```python
from build123d import *

# Parameters (mm, degrees)
CROQUIS1_W              = 160
CROQUIS1_H              = 50.8
SALIENTE_EXTRUIR1_DEPTH = 300
CROQUIS2_W              = 160
CROQUIS2_H              = 25.4
SALIENTE_EXTRUIR2_DEPTH = 100
CROQUIS3_R              = 12.5
CORTAR_EXTRUIR1_DEPTH   = 100
CROQUIS4_R              = 18
CORTAR_EXTRUIR2_DEPTH   = 5
CORTAR_EXTRUIR3_START   = -5
CROQUIS5_R              = 18
CORTAR_EXTRUIR3_DEPTH   = 5


with BuildPart() as part:
    # Croquis1 → Saliente-Extruir1 (new, symmetric)
    with BuildSketch(Plane.XY):
        Rectangle(CROQUIS1_W, CROQUIS1_H)
    extrude(amount=SALIENTE_EXTRUIR1_DEPTH, both=True)

    # Croquis2 → Saliente-Extruir2 (add)
    with BuildSketch(Plane(origin=(0, 25.4, 0), x_dir=(1, 0, 0), z_dir=(0, 1, 0))):
        with Locations((0, 287.3)):
            Rectangle(CROQUIS2_W, CROQUIS2_H)
    extrude(amount=SALIENTE_EXTRUIR2_DEPTH)

    # Croquis3 → Cortar-Extruir1 (cut)
    with BuildSketch(Plane.XY.offset(-274.6)):
        with Locations((0, 59.234859244)):
            Circle(CROQUIS3_R)
    extrude(amount=-CORTAR_EXTRUIR1_DEPTH, mode=Mode.SUBTRACT)

    # Croquis4 → Cortar-Extruir2 (cut)
    with BuildSketch(Plane.XY.offset(-274.6)):
        with Locations((0, 59.234859244)):
            Circle(CROQUIS4_R)
    extrude(amount=-CORTAR_EXTRUIR2_DEPTH, mode=Mode.SUBTRACT)

    # Croquis5 → Cortar-Extruir3 (cut)
    with BuildSketch(Plane(origin=(0, 0, -300), x_dir=(-1, 0, 0), z_dir=(0, 0, -1)).offset(CORTAR_EXTRUIR3_START)):
        with Locations(Location((0, 59.234859244, 0), (0, 0, 180))):
            Circle(CROQUIS5_R)
    extrude(amount=CORTAR_EXTRUIR3_DEPTH, mode=Mode.SUBTRACT)


solid = part.part
```
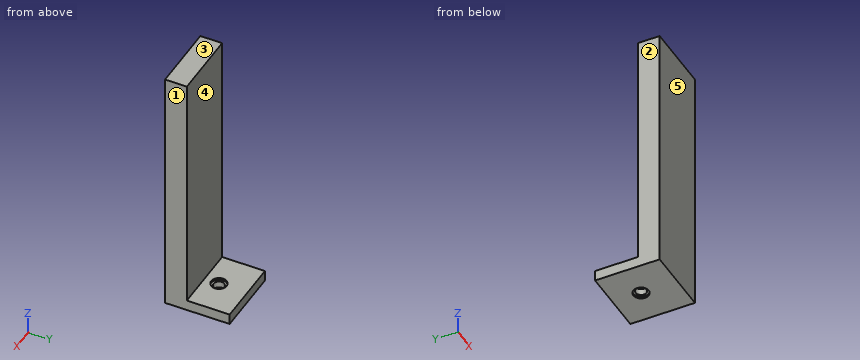
Verification items for the finished model (mm, model axes). Face numbers are marked on the shaded views. A direction names the side the tool comes from. Give positions to 0.01 mm unless a question says otherwise; leave off trailing zeros. Order: outer loops, then holes, each group sorted by start corner. A loop starts at its lowest first (then second) coordinate and runs counter-clockwise, first axis right, second up. Notation, with made-up numbers: (30, -17) -> (79, -17) arc R11 ccw to (79, -13) -> close; hole circle Ø4 at (-8.75, -21). An arc over 180 degrees is marked (long way). Use a Markdown table: item, result.
1) Section check A-A, the plane x = 0. Record the boundary of the cut face in (y, z), then the cut area to 3 significant figures.
Results:
| item | result |
|---|---|
| outline | (-25.4, -300) -> (41.23, -300) -> (41.23, -295) -> (46.73, -295) -> (46.73, -279.6) -> (41.23, -279.6) -> (41.23, -274.6) -> (25.4, -274.6) -> (25.4, 300) -> (-25.4, 300) -> close; (71.73, -295) -> (77.23, -295) -> (77.23, -300) -> (125.4, -300) -> (125.4, -274.6) -> (77.23, -274.6) -> (77.23, -279.6) -> (71.73, -279.6) -> close |
| area | 32,300 mm² |
2) Material ranges on probe 1 along Y at (x, z) = (0, -285.75); probe 2 along Y at (x, z) = (0, -277); probe 3 along Y at (x, z) = (13.5, 67.5), recorded low to high.
Results:
| item | result |
|---|---|
| probe 1 | -25.4 to 46.73, 71.73 to 125.4 |
| probe 2 | -25.4 to 41.23, 77.23 to 125.4 |
| probe 3 | -25.4 to 25.4 |
3) Tool access check on the marked faces 4 and 5. Record the directions out of +Z, -Z, +X, -X, +Y, -Y that give a thin tool (end or side, any length) a straight path to the whole face; none if there is none.
Results:
| item | result |
|---|---|
| face 4 | +Z, +X, -X, +Y |
| face 5 | +Z, -Z, +X, -X, -Y |
4) Section check D-D, the plane z = 167.5. Record the boundary of the cut face in (x, y).
Results:
| item | result |
|---|---|
| outline | (-80, -25.4) -> (80, -25.4) -> (80, 25.4) -> (-80, 25.4) -> close |
5) Section check C-C, the plane y = 100. Record the boundary of the cut face in (x, z).
Results:
| item | result |
|---|---|
| outline | (-80, -300) -> (80, -300) -> (80, -274.6) -> (-80, -274.6) -> close |
6) Mould release check, pull along X, two halves, no side actions. Record for the marked faces 1, 2 and 3: pulls with the +X half, pulls with the -X half, needs draft (parallel to the pull), parting line crosses it, or undercut.
Results:
| item | result |
|---|---|
| face 1 | pulls with the +X half |
| face 2 | pulls with the -X half |
| face 3 | needs draft |
7) Section check B-B, the plane x = -39.5. Record the boundary of the cut face in (y, z), then the cut area to 3 significant figures.
Results:
| item | result |
|---|---|
| outline | (-25.4, -300) -> (125.4, -300) -> (125.4, -274.6) -> (25.4, -274.6) -> (25.4, 300) -> (-25.4, 300) -> close |
| area | 33,000 mm² |
8) Depth check by flat-ended pin: pin 1 Ø1 at (x, z) = (26.5, 12) entering from +Y; pin 2 Ø18 at (x, y) = (-3, 66) entering from +Z; pin 3 Ø18 at (x, y) = (2, 54) entering from -Z. Enter the tip coordinate at first touch or a pass-through.
Results:
| item | result |
|---|---|
| pin 1 | y = 25.4 |
| pin 2 | z = -279.6 |
| pin 3 | z = -295 |
